Part model, mm, in its own coordinate system. Face numbers are marked on the shaded views. A direction names the side the tool comes from. Give positions to 0.01 mm unless a question says otherwise; leave off trailing zeros. Loops run counter-clockwise (first coordinate to the right, second up) from the corner with the lowest first, then second, coordinate; pieces in that order, holes last. Notation, with made-up numbers: (54.5, 40.25) -> (61.5, 40.25) arc R17 ccw to (61.5, 65.25) -> close; hole circle Ø9 at (6, 50.5). An arc over 180 degrees is marked (long way). Write item = value, one per line.
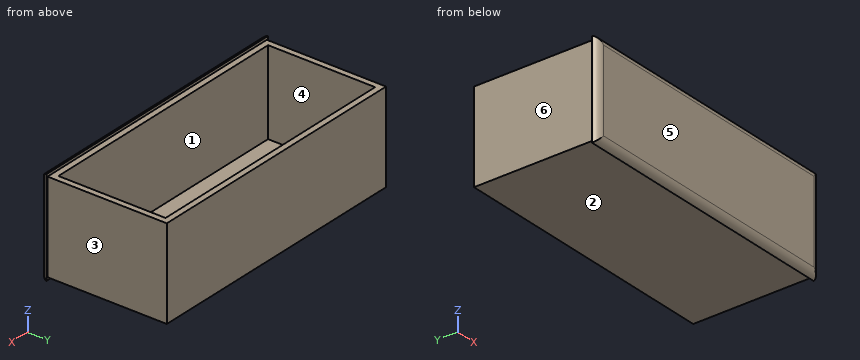
from build123d import *

# Parameters (mm, degrees)
F0_W        = 580.39
F0_H        = 250.19
F1_DEPTH    = 95.25
F2_T        = -12.7
F3_W        = 542.29
F3_H        = 171.45
F4_DEPTH    = 25.4
F5_W        = 586.74
F5_H        = 201.93
F6_DEPTH    = 12.7
F7_T1_DEPTH = 661.8742132454
F7_T3_DEPTH = 277.0642132454
F8_DEPTH    = 171.45


# Not quite as in the source:
# - a fillet or chamfer that OpenCascade refuses, or shapes differently, is made with other operations: its cross-section is extruded or revolved along the edge and cut away or added


with BuildPart() as f1:
    # F0 (on Top) → F1 (new body, symmetric)
    with BuildSketch(Plane.XY):
        Rectangle(F0_W, F0_H)
    extrude(amount=F1_DEPTH, both=True)

    # F2
    f2_openings = [f1.faces().sort_by_distance(p)[0] for p in [
        (0, 0, 95.25),
    ]]
    offset(amount=F2_T, openings=f2_openings)

    # F3 (on face) → F4 (cut)
    with BuildSketch(Plane.XZ.offset(125.095)):
        with Locations((0, 9.525)):
            Rectangle(F3_W, F3_H)
    extrude(amount=-F4_DEPTH, mode=Mode.SUBTRACT)

    # F5 (on face) → F6 (join)
    with BuildSketch(Plane.XZ.offset(125.095)):
        Rectangle(F5_W, F5_H)
        Polygon((-290.195, -95.25), (-290.195, 95.25), (-271.145, 95.25), (-271.145, -76.2), (271.145, -76.2), (271.145, 95.25), (290.195, 95.25), (290.195, -95.25), align=None, mode=Mode.SUBTRACT)
        Polygon((-271.145, 95.25), (-290.195, 95.25), (-290.195, -95.25), (290.195, -95.25), (290.195, 95.25), (271.145, 95.25), (271.145, -76.2), (-271.145, -76.2), align=None)
    extrude(amount=F6_DEPTH)

    # F7: fillet of radius 15.24 on 4 edges, made by hand

    # F7_s2 → F7_t1 (cut)
    with BuildSketch(Plane.YZ.offset(-330.9371066227)):
        with BuildLine():
            ThreePointArc((-125.095, 100.965), (-134.1947422652, 95.7755350503), (-137.795, 85.9381573509))
            Line((-137.795, 85.9381573509), (-137.795, 100.965))
            Line((-137.795, 100.965), (-125.095, 100.965))
        make_face()
        with BuildLine():
            ThreePointArc((-125.095, -100.965), (-134.1947422652, -95.7755350503), (-137.795, -85.9381573509))
            Line((-137.795, -85.9381573509), (-137.795, -100.965))
            Line((-137.795, -100.965), (-125.095, -100.965))
        make_face()
    extrude(amount=F7_T1_DEPTH, mode=Mode.SUBTRACT)

    # F7_s4 → F7_t3 (cut)
    with BuildSketch(Plane.XY.offset(-138.5321066227)):
        with BuildLine():
            ThreePointArc((-278.3431573509, -137.795), (-288.1805350503, -134.1947422652), (-293.37, -125.095))
            Line((-293.37, -125.095), (-293.37, -137.795))
            Line((-293.37, -137.795), (-278.3431573509, -137.795))
        make_face()
        with BuildLine():
            ThreePointArc((293.37, -125.095), (288.1805350503, -134.1947422652), (278.3431573509, -137.795))
            Line((278.3431573509, -137.795), (293.37, -137.795))
            Line((293.37, -137.795), (293.37, -125.095))
        make_face()
    extrude(amount=F7_T3_DEPTH, mode=Mode.SUBTRACT)

    # F8 (add): a face of the model
    f8_faces = [f1.faces().sort_by_distance(p)[0] for p in [
        (0, -118.745, -76.2),
    ]]
    extrude(f8_faces, amount=F8_DEPTH)


solid = f1.part
1) Slice it at B-B, the plane y = 31.5. List the corners of the cut face in (x, z) (3 decimals).
Resolved:
outline = (-290.195, -95.25) -> (290.195, -95.25) -> (290.195, 95.25) -> (277.495, 95.25) -> (277.495, -82.55) -> (-277.495, -82.55) -> (-277.495, 95.25) -> (-290.195, 95.25) -> close
2) Slice it at A-A, the plane z = -63. List the corners of the cut face in (x, y) (3 decimals).
Resolved:
outline = (-293.37, -125.095) arc R15.24 ccw to (-278.343, -137.795) -> (278.343, -137.795) arc R15.24 ccw to (293.37, -125.095) -> (290.195, -125.095) -> (290.195, 125.095) -> (-290.195, 125.095) -> (-290.195, -125.095) -> close; hole (-277.495, -112.395) -> (277.495, -112.395) -> (277.495, 112.395) -> (-277.495, 112.395) -> close
3) Which spindle directions (+Z, -Z, +X, -X, +Y, -Y) get a long thin tool onto all of the face, cutting with end or side? Do the marked faces 5 and 6. Say none if no direction does.
Resolved:
face_5 = +Z, -Z, +X, -X, -Y
face_6 = +Z, -Z, -X, +Y
4) Slice it at C-C, the plane x = -76. List the corners of the cut face in (y, z) (3 decimals), and give its area (3 significant figures).
Resolved:
outline = (-137.795, -85.938) arc R15.24 ccw to (-125.095, -100.965) -> (-125.095, -95.25) -> (125.095, -95.25) -> (125.095, 95.25) -> (112.395, 95.25) -> (112.395, -82.55) -> (-112.395, -82.55) -> (-112.395, 95.25) -> (-125.095, 95.25) -> (-125.095, 100.965) arc R15.24 ccw to (-137.795, 85.938) -> close
area = 10,200 mm²
5) Drill centre lines: line 1 along Y through (x, z) = (-10, -8) (3 decimals); line 2 along X through (y, z) = (-19, 75) (3 decimals); line 3 along Z through (x, y) = (204.5, -5.5). Where is each one in solid material? Low to high. Write a range as [from, to].
Resolved:
line_1 = [-137.795, -112.395], [112.395, 125.095]
line_2 = [-290.195, -277.495], [277.495, 290.195]
line_3 = [-95.25, -82.55]
6) Pull direction X, two halves, no side cores. Call the marked faces 1, 2, 3 and 4: pulls with the +X half, pulls with the -X half, needs draft (parallel to the pull), parting line crosses it, or undercut.
Resolved:
face_1 = undercut
face_2 = needs draft
face_3 = pulls with the +X half
face_4 = undercut
7) Drop flat-ended pins along their axis: P1, Ø4, axis at y = -85.5, z = 5, coming from the +X side (3 decimals); P2, Ø3, axis at x = -10, y = 51, coming from the -Z side; P3, Ø5, axis at y = 34.5, z = 23, coming from the -X side (3 decimals). Give the stop position or say it passes through.
Resolved:
P1 = 290.195
P2 = -95.25
P3 = -290.195
